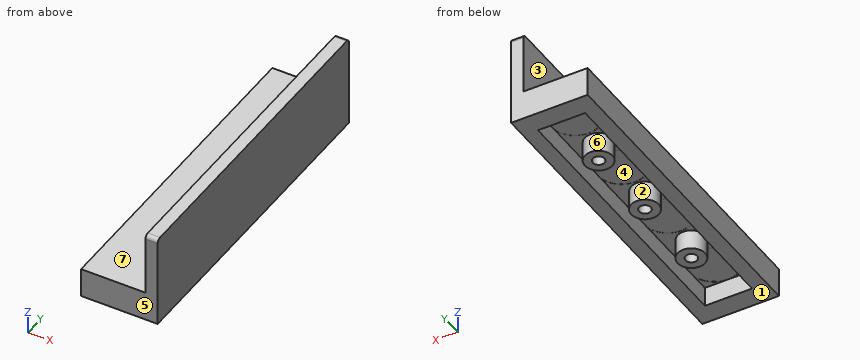
Solid Edge part; units mm, degrees
sketch "Sketch1" plane through (0, 0, 0) normal (0, -1, 0) x (1, 0, 0)
  line L0 (0, 3) -> (6.55, 3)
  line L1 (6.55, 9.4) -> (6.55, 3)
  line L2 (7.8, 9.4) -> (6.55, 9.4)
  line L3 (7.8, 0) -> (7.8, 9.4)
  line L4 (0, 0) -> (7.8, 0)
  line L5 (0, 3) -> (0, 0)
extrude "Protrusion1" add sketch "Sketch1" against normal blind 33
sketch "Sketch2" plane through (3.9, 16.5, 0) normal (0, 0, -1) x (0, -1, 0)
  line L0 (-14.4, -2.4) -> (14.4, -2.4)
  line L1 (14.4, -2.4) -> (14.4, 2.4)
  line L2 (14.4, 2.4) -> (-14.4, 2.4)
  line L3 (-14.4, 2.4) -> (-14.4, -2.4)
  circle A0 centre (-8, 0) radius 1.4
  circle A1 centre (0, 0) radius 1.4
  circle A2 centre (8, 0) radius 1.4
  circle A3 centre (-8, 0) radius 0.6
  circle A4 centre (0, 0) radius 0.6
  circle A5 centre (8, 0) radius 0.6
extrude "ExtrudedCutout_1" cut sketch "Sketch2" against normal blind 2
fillet "Round_1" radius 0.4 2 edges at (7.175, 33, 9.4) (7.175, 0, 9.4)
sketch "Sketch3" plane through (3.9, 16.5, 2) normal (0, 0, -1) x (0, -1, 0)
  circle A0 centre (-12, -0.053) radius 2.4
  circle A1 centre (-4, -0.053) radius 2.4
  circle A2 centre (4, -0.053) radius 2.4
  circle A3 centre (12, -0.053) radius 2.4
extrude "ExtrudedCutout_2" cut sketch "Sketch3" against normal blind 0.01
Build history of the part. All positions in model axes, mm. Face numbers are marked on the shaded views. A direction names the side the tool comes from. Round coordinates to 2 decimals unless told otherwise and drop trailing zeros. Loops run counter-clockwise (first coordinate to the right, second up) from the corner with the lowest first, then second, coordinate; pieces in that order, holes last. Notation, with made-up numbers: (-6.5, 39.25) -> (43.5, 39.25) arc R19 ccw to (43.5, 57.25) -> close; hole circle Ø7 at (86, -8). An arc over 180 degrees is marked (long way). Answer in a Markdown table with one row per item.
Item 1: Saw through at B-B (z = 5). Write the cut outline in (x, y).
Answers below:
| item | result |
|---|---|
| outline | (6.55, 0) -> (7.8, 0) -> (7.8, 33) -> (6.55, 33) -> close |
Item 2: Saw through at D-D (y = 16.5). Write the cut outline in (x, z), and give its area (3 significant figures).
Answers below:
| item | result |
|---|---|
| outline | (0, 0) -> (1.5, 0) -> (1.5, 2) -> (2.5, 2) -> (2.5, 0) -> (3.3, 0) -> (3.3, 2) -> (4.5, 2) -> (4.5, 0) -> (5.3, 0) -> (5.3, 2) -> (6.3, 2) -> (6.3, 0) -> (7.8, 0) -> (7.8, 9.4) -> (6.55, 9.4) -> (6.55, 3) -> (0, 3) -> close |
| area | 25.0 mm² |
Item 3: Pin check, flat tips, straight feed: pin 1 (1.4 mm diameter, centred on x = 3, y = 12, fed in from -Z); pin 2 (5 mm diameter, centred on y = 18, z = 6.5, fed in from -X); pin 3 (1 mm diameter, centred on x = 1.5, y = 18, fed in from +Z). Stop position of each tip, or through.
Answers below:
| item | result |
|---|---|
| pin 1 | stops at z = 2.01 |
| pin 2 | stops at x = 6.55 |
| pin 3 | stops at z = 3 |
Item 4: Mould opens along Y. For the marked faces 4, 5, 6 and 7 say: +Y half, -Y half, draft (parallel to the pull), parting line (faces both ways), or undercut.
Answers below:
| item | result |
|---|---|
| face 4 | undercut |
| face 5 | -Y half |
| face 6 | undercut |
| face 7 | draft |
Item 5: Which spindle directions (+Z, -Z, +X, -X, +Y, -Y) get a long thin tool onto all of the face, cutting with end or side? Do the marked faces 1, 2 and 3. Say none if no direction does.
Answers below:
| item | result |
|---|---|
| face 1 | -Z, +X, -X, +Y, -Y |
| face 2 | -Z |
| face 3 | +Z, -X, +Y, -Y |
Item 6: Drill centre lines: L1, parallel to X at y = 16.5, z = 1; L2, parallel to X at y = 29.5, z = 0.5; L3, parallel to X at y = 15, z = 5. Where is each one in solid material? Low to high. Write a range as [from, to].
Answers below:
| item | result |
|---|---|
| L1 | x = [0, 1.5], [2.5, 3.3], [4.5, 5.3], [6.3, 7.8] |
| L2 | x = [0, 1.5], [6.3, 7.8] |
| L3 | x = [6.55, 7.8] |
